```python
from build123d import *

# Parameters (mm, degrees)
F0_R     = 12.7
F1_DEPTH = 152.4
F2_R     = 76.19999
F3_R     = 38.1
F4_DEPTH = 42.1602994648
F3_W     = 101.6
F3_H     = 25.4
F5_DEPTH = 42.1602994648
F7_DEPTH = 45.29165
F9_DEPTH = 152.401


# Not quite as in the source:
# - a fillet or chamfer is up to 0.001 mm smaller than in the source, because OpenCascade refuses the exact size


with BuildPart() as f1:
    # F0 (on Front) → F1 (new body)
    with BuildSketch(Plane.XZ):
        with BuildLine():
            ThreePointArc((12.2889600906, 43.2626888076), (-4.7984134102, 87.7468446554), (-20.7310399094, 42.83615698))
            Line((-20.7310399094, 42.83615698), (-20.7310399094, -140.8510365048))
            Line((-20.7310399094, -140.8510365048), (12.2889600906, -140.8510365048))
            Line((12.2889600906, -140.8510365048), (12.2889600906, 43.2626888076))
        make_face()
        with Locations((-4.4703393742, 62.3489634952)):
            Circle(F0_R, mode=Mode.SUBTRACT)
    extrude(amount=F1_DEPTH)

    # F2 (radius 76.2 in the source; OpenCascade refuses exactly that, so slightly less here)
    f2_edges = [f1.edges().sort_by_distance(p)[0] for p in [
        (-4.22104, -152.4, -140.851037),
        (-4.22104, 0, -140.851037),
    ]]
    fillet(f2_edges, radius=F2_R)

    # F3 (on face) → F4 (cut, through all)
    with BuildSketch(Plane.YZ.offset(12.2889600906)):
        with Locations((-76.2, -64.6510365048)):
            Circle(F3_R)
    extrude(amount=-F4_DEPTH, mode=Mode.SUBTRACT)

    # F3 (on face) → F5 (cut, through all)
    with BuildSketch(Plane.YZ.offset(12.2889600906)):
        with Locations((-76.2, 30.5626888076)):
            Rectangle(F3_W, F3_H)
    extrude(amount=-F5_DEPTH, mode=Mode.SUBTRACT)

    # F6 (on face) → F7 (cut, symmetric)
    with BuildSketch(Plane(origin=(-20.7310399094, 0, 0), x_dir=(0, -1, 0), z_dir=(-1, 0, 0))):
        Polygon((25.4293922335, 17.8626888076), (127, 17.8626888076), (127, 42.83615698), (127, 109.7837612033), (25.4293922335, 109.7837612033), align=None)
    extrude(amount=F7_DEPTH, both=True, mode=Mode.SUBTRACT)

    # F8 (on face) → F9 (cut, through all)
    with BuildSketch(Plane.XZ.offset(152.4)):
        with BuildLine():
            Line((0, -32.9373111924), (0, 17.8626878918))
            ThreePointArc((0, 17.8626878918), (-6.35, 24.2126888076), (-12.7, 17.8626878918))
            Line((-12.7, 17.8626878918), (-12.7, -32.9373111924))
            ThreePointArc((-12.7, -32.9373111924), (-6.35, -39.2873111924), (0, -32.9373111924))
        make_face()
    extrude(amount=-F9_DEPTH, mode=Mode.SUBTRACT)


solid = f1.part
```
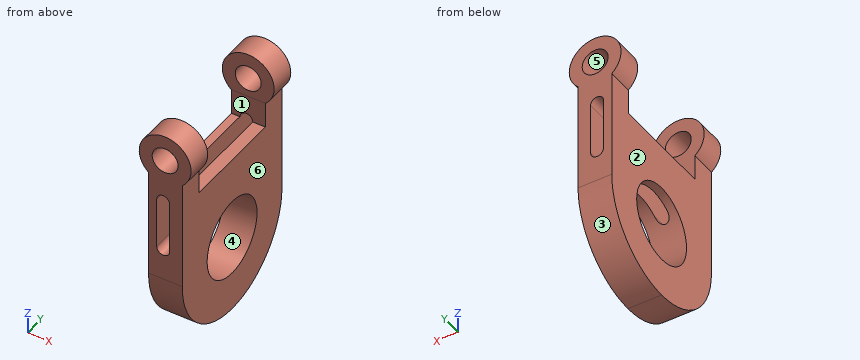
Geometry: final body of the model. Coordinates: model frame, mm. Face numbers are marked on the shaded views. A direction names the side the tool comes from. Round coordinates to 2 decimals unless told otherwise and drop trailing zeros. Order: outer loops, then holes, each group sorted by start corner. A loop starts at its lowest first (then second) coordinate and runs counter-clockwise, first axis right, second up. Notation, with made-up numbers: M -5,-33 L 5,-33 A22 cw 5,3 Z; hole C -1.5,-19 d4. An arc over 180 degrees is marked long. Use one line per item in the form item = value. Start each with the question number.
Q1. Cut plane A-A (z = 32). Return loops of the section in (x, y).
Q2. Material intervals for line 1 (X direction, y = -127, z = -7.5); line 2 (Y direction, x = 12, z = 59); line 3 (X direction, y = -20.5, z = -94), sorted ascending. Write a range as [from, to].
Q3. Mould query, pull axis Y, two halves, no side actions, for the marked faces 1, 2, 3 and 4. Classes: +Y half, -Y half, draft (parallel to the pull), parting line (faces both ways), or undercut.
Q4. Pin query (flat end, axial travel): pin 1 Ø20.5 at (x, z) = (-4.47, 62.35) entering from +Y; pin 2 Ø6 at (x, y) = (-9, -50) entering from -Z; pin 3 Ø6 at (y, z) = (-134, 20.5) entering from +X; pin 4 Ø2.5 at (x, y) = (-17, -72.5) entering from +Z. Return the tip coordinate at first contact, or that it passes through.
Q5. Cut plane D-D (x = 15). Return loops of the section in (y, z), and give its area (3 significant figures).
Q6. Access query for the marked faces 5 and 6. Directions: +Z, -Z, +X, -X, +Y, -Y. A direction counts if a zero-diameter tool reaches every point of the face in a straight line with its end or side. Return the directions, or none.
Q7. Cut plane B-B (x = -6.35). Count the separate pieces of the cut face and the enclosed holes in it, and give its area (3 significant figures).
Geometry results:
q1.outline = M -20.73,-152.4 L 12.29,-152.4 L 12.29,-127 L -20.73,-127 Z; M -20.73,-25.4 L 12.29,-25.4 L 12.29,0 L -20.73,0 Z
q2.line_1 = [-20.73, -12.7], [0, 12.29]
q2.line_2 = [-152.4, -127], [-25.43, 0]
q2.line_3 = [-20.73, 12.29]
q3.face_1 = undercut
q3.face_2 = draft
q3.face_3 = +Y half
q3.face_4 = undercut
q4.pin_1 = through
q4.pin_2 = -137.23
q4.pin_3 = 12.29
q4.pin_4 = 17.86
q5.outline = M -152.4,46.04 L -127,46.04 L -127,78.66 L -152.4,78.66 Z; M -25.43,46.04 L 0,46.04 L 0,78.66 L -25.43,78.66 Z
q5.area = 1,660 mm^2
q6.face_5 = +Y, -Y
q6.face_6 = -Z, +X, +Y, -Y
q7.separate_pieces = 5
q7.enclosed_holes = 0
q7.area = 10,900 mm^2
